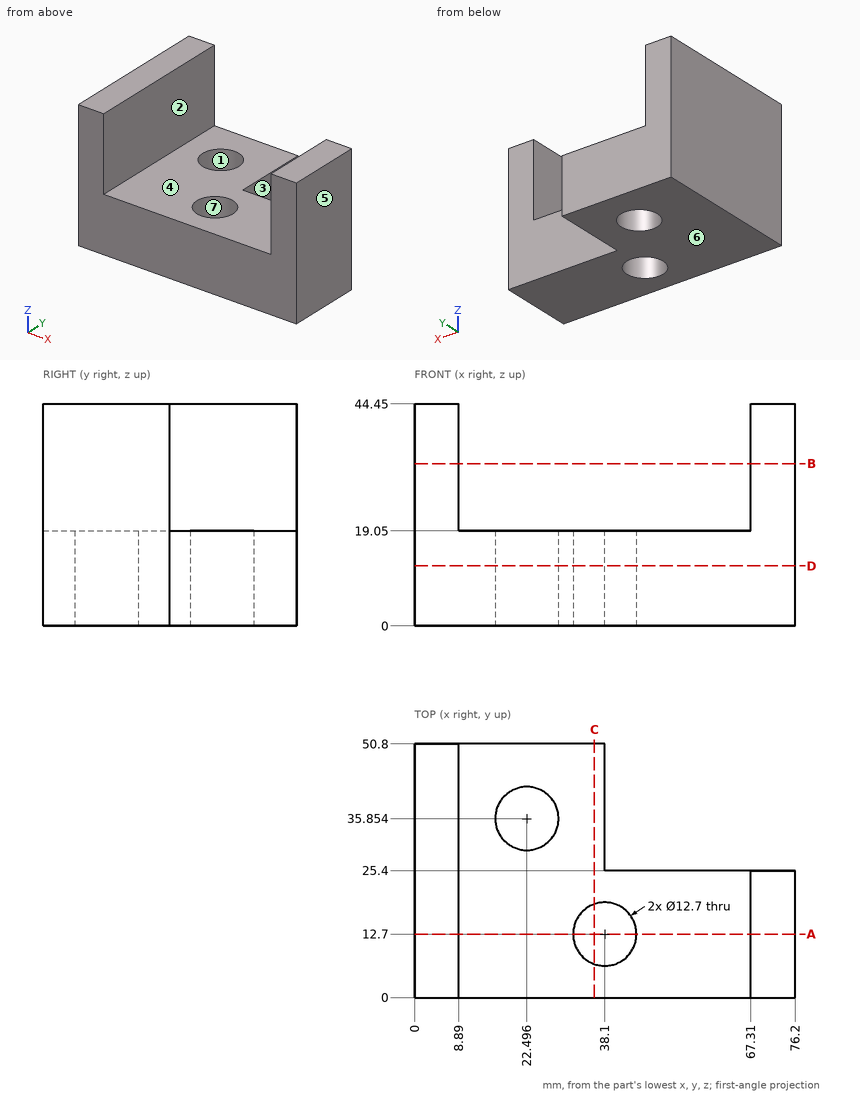
Drawing for the job (mm, zero at the part's lowest x, y, z). A direction names the side the tool comes from. Round coordinates to 2 decimals unless told otherwise and drop trailing zeros. Write each loop counter-clockwise with the first axis right and the second up, starting at its lowest first coordinate (ties: lowest second). Pieces come first, ordered by that corner, then holes.
Item 1: Band-saw the part on D-D on z = 12. Give the number of separate pieces and of enclosed holes in the cut face, then the cut area to 3 significant figures.
Filled in:
separate pieces: 1
enclosed holes: 2
area: 2,650 mm2
Item 2: Band-saw the part on B-B on z = 32.5. Write the cut outline in (x, y).
Filled in:
outline: (0, 0) - (8.89, 0) - (8.89, 50.8) - (0, 50.8) - close; (67.31, 0) - (76.2, 0) - (76.2, 25.4) - (67.31, 25.4) - close
Item 3: Mould opens along X. For the marked faces 4, 5, 6 and 7 say: released by +X, released by -X, zero draft, split by the parting line, or undercut.
Filled in:
face 4: undercut
face 5: released by +X
face 6: zero draft
face 7: undercut
Item 4: Band-saw the part on C-C on x = 36. Write the cut outline in (y, z).
Filled in:
outline: (0, 0) - (6.71, 0) - (6.71, 19.05) - (0, 19.05) - close; (18.69, 0) - (50.8, 0) - (50.8, 19.05) - (18.69, 19.05) - close
Item 5: Band-saw the part on A-A on y = 12.7. Write the cut outline in (x, z).
Filled in:
outline: (0, 0) - (31.75, 0) - (31.75, 19.05) - (8.89, 19.05) - (8.89, 44.45) - (0, 44.45) - close; (44.45, 0) - (76.2, 0) - (76.2, 44.45) - (67.31, 44.45) - (67.31, 19.05) - (44.45, 19.05) - close
Item 6: Tool access for the marked faces 1, 2 and 3: list every direction of +Z, -Z, +X, -X, +Y, -Y with a clear straight run to the whole face (end or side of a thin tool).
Filled in:
face 1: +Z, -Z
face 2: +Z, +Y, -Y
face 3: +Z, -Z, +X, +Y
Item 7: Drop flat-ended pins along their axis: pin 1 Ø1 at (x, y) = (30, 9) entering from -Z; pin 2 Ø16.5 at (x, y) = (38.1, 12.7) entering from +Z; pin 3 Ø9.5 at (y, z) = (34, 11) entering from +X; pin 4 Ø19 at (x, z) = (50, 31.5) entering from +Y. Give the stop position or say it passes through.
Filled in:
pin 1: stops at z = 0
pin 2: stops at z = 19.05
pin 3: stops at x = 38.1
pin 4: passes through
Item 8: Drill centre lines: L1, parallel to Y at x = 38, z = 10; L2, parallel to Z at x = 16, y = 6; L3, parallel to X at y = 5, z = 26.5. Where is each one in solid material? Low to high.
Filled in:
L1: y = 0 to 6.35, 19.05 to 50.8
L2: z = 0 to 19.05
L3: x = 0 to 8.89, 67.31 to 76.2
